```python
from build123d import *

# Parameters (mm, degrees)
EXTRUDE1_DEPTH       = 0.8
EXTRUDE2_DEPTH       = 5.5
DRAFT1_ANGLE         = -33.206570315
DRAFT2_ANGLE         = -33.206570315
M6_CLEARANCE_HOLE1_D = 7
CHAMFER1_SIZE        = 0.433


with BuildPart() as part:
    # Sketch1 → Extrude1 (new body)
    with BuildSketch(Plane(origin=(0, 0, 0), x_dir=(0, 0, -1), z_dir=(1, 0, 0))):
        with BuildLine():
            Line((1.101052702, 3.9), (-5.186106572, 3.9))
            Line((-5.186106572, 3.9), (-3.612459851, -1.972929517))
            ThreePointArc((-3.612459851, -1.972929517), (-2.683832418, -3.362718685), (-1.101052702, -3.9))
            Line((-1.101052702, -3.9), (5.186106572, -3.9))
            Line((5.186106572, -3.9), (3.612459851, 1.972929517))
            ThreePointArc((3.612459851, 1.972929517), (2.683832418, 3.362718685), (1.101052702, 3.9))
        make_face()
    extrude(amount=-EXTRUDE1_DEPTH)

    # Sketch2 → Extrude2 (add)
    with BuildSketch(Plane.ZY.offset(0.8)):
        with BuildLine():
            Line((2.131485778, -7.5), (-6.150723665, -7.5))
            add(Edge.make_bspline(
                [(-2.131485778, 7.5), (-3.471231741, 2.5), (-4.810977703, -2.5), (-6.150723665, -7.5)],
                knots=[0, 0, 0, 0, 1, 1, 1, 1], degree=3))
            Line((-2.131485778, 7.5), (6.150723665, 7.5))
            add(Edge.make_bspline(
                [(2.131485778, -7.5), (3.471231741, -2.5), (4.810977703, 2.5), (6.150723665, 7.5)],
                knots=[0, 0, 0, 0, 1, 1, 1, 1], degree=3))
        make_face()
    extrude(amount=EXTRUDE2_DEPTH)

    # Draft1
    draft1_faces = [part.faces().sort_by_distance(p)[0] for p in [
        (-3.55, 7.5, 2.009618943),
    ]]
    draft(draft1_faces, Plane(origin=(-0.8, 0, 4.141104722), x_dir=(0, 0, 1), z_dir=(1, 0, 0)), DRAFT1_ANGLE)

    # Draft2
    draft2_faces = [part.faces().sort_by_distance(p)[0] for p in [
        (-3.55, -7.5, -2.009618943),
    ]]
    draft(draft2_faces, Plane(origin=(-0.8, 0, 4.141104722), x_dir=(0, 0, 1), z_dir=(1, 0, 0)), DRAFT2_ANGLE)

    # M6 Clearance Hole1 (through all)
    with Locations(Plane.ZY.offset(6.3)):
        with Locations((0, 0)):
            Hole(M6_CLEARANCE_HOLE1_D / 2)

    # Chamfer1
    # the kernel refuses this chamfer: 0.433 mm, written as the material it takes off along each edge
    with BuildSketch(Plane(origin=(0, 0, 0), x_dir=(0, 0, -1), z_dir=(0, -1, 0))) as chamfer1_piece_1:
        Polygon((3.5 + CHAMFER1_SIZE, 0), (3.5, -CHAMFER1_SIZE), (3.5, 0), align=None)
    revolve(axis=Axis((0, 0, 0), (1, 0, 0)), mode=Mode.SUBTRACT)
    with BuildSketch(Plane(origin=(-6.3, 0, 0), x_dir=(0, 0, -1), z_dir=(0, -1, 0))) as chamfer1_piece_2:
        Polygon((3.5 + CHAMFER1_SIZE, 0), (3.5, CHAMFER1_SIZE), (3.5, 0), align=None)
    revolve(axis=Axis((-6.3, 0, 0), (1, 0, 0)), mode=Mode.SUBTRACT)


solid = part.part
```
Build history of the part. All positions in model axes, mm. A direction names the side the tool comes from. Give positions to 0.01 mm unless a question says otherwise; leave off trailing zeros. Order: outer loops, then holes, each group sorted by start corner. A loop starts at its lowest first (then second) coordinate and runs counter-clockwise, first axis right, second up. Notation, with made-up numbers: M 37,76.25 L 91,76.25 A35 ccw 91,108.25 Z; hole C 19,26 d1. An arc over 180 degrees is marked long. Return JSON: item names as keys, results as strings.
Q1. Flat gauge pins, fed straight in: pin 1 (1.5 mm diameter, centred on x = -3.5, y = 1, fed in from +Z); pin 2 (3 mm diameter, centred on y = 6, z = 2.5, fed in from +X); pin 3 (3 mm diameter, centred on x = -3.5, z = 3, fed in from -Y). Where does each tip first touch, or does it go through?
Answer list:
{"pin 1": "stops at z = 4.61", "pin 2": "stops at x = -0.8", "pin 3": "stops at y = -6.62"}
Q2. Wall check: probe 1 along X at (y, z) = (-3.25, 3); probe 2 along Y at (x, z) = (-2.7, 0); probe 3 along Z at (x, y) = (-3.5, -1.75). Give the ranges that are in metal, low to high. Write a range as from..to.
Answer list:
{"probe 1": "x = -6.3..-0.8", "probe 2": "y = -6.26..-3.5, 3.5..6.26", "probe 3": "z = -4.61..-3.03, 3.03..3.67"}
Q3. 3-axis set-ups, long thin cutter, end or side, ignore diameter. For faces 4 (the face through (-0.39, 3.35, -2.7)), 5 (the face through (-0.4, -3.9, -2)), 6 (the face through (-0.39, -3.35, 2.7)): which of +Z, -Z, +X, -X, +Y, -Y reach the whole face in a straight line?
Answer list:
{"face 4": "-Z, +X, +Y", "face 5": "+Z, -Z, +X, -Y", "face 6": "+Z, +X, -Y"}
Q4. Two-plate mould, pull along Z, no slides. Class faces 1 (the face through (-3.112, -1.341, -3.233)), 2 (the face through (-0.39, 1, 4.41)), 3 (the face through (-0.4, 3.9, 2)): pulls with the +Z half, pulls with the -Z half, needs draft (parallel to the pull), parting line crosses it, or undercut.
Answer list:
{"face 1": "undercut", "face 2": "pulls with the +Z half", "face 3": "needs draft"}
Q5. Band-saw the part on A-A (z = 0). Give the cut face in (x, y).
Answer list:
{"outline": "M -6.28,-3.91 L -0.8,-7.5 L -0.8,-3.9 L -0.03,-3.9 L -0.43,-3.5 L -5.87,-3.5 Z; M -6.28,3.91 L -5.87,3.5 L -0.43,3.5 L -0.03,3.9 L -0.8,3.9 L -0.8,7.5 Z"}
